```python
from build123d import *

# Parameters (mm, degrees)
F1_DEPTH = 15
F2_R     = 2.125
F3_DEPTH = 18.001
F4_R     = 3.5
F5_DEPTH = 6


with BuildPart() as f1:
    # F0 (on Top) → F1 (new body)
    with BuildSketch(Plane.XY):
        with BuildLine():
            Line((-13.829164, 6.4), (-13.829164, 0))
            Line((-13.829164, 0), (20, 0))
            Line((20, 0), (20, 5))
            Line((20, 5), (10, 5))
            Line((10, 5), (10, 8))
            ThreePointArc((10, 8), (7.071068, 15.071068), (0, 18))
            Line((0, 18), (-13.829164, 18))
            Line((-13.829164, 18), (-13.829164, 9.6))
            Line((-13.829164, 9.6), (-3.829164, 9.6))
            ThreePointArc((-3.829164, 9.6), (4.15, 8), (-3.829164, 6.4))
            Line((-3.829164, 6.4), (-13.829164, 6.4))
        make_face()
    extrude(amount=F1_DEPTH)

    # F2 (on face) → F3 (cut, through all)
    with BuildSketch(Plane.XZ):
        with Locations((-7.5, 7.5)):
            Circle(F2_R)
        with Locations((15, 7.5)):
            Circle(F2_R)
    extrude(amount=-F3_DEPTH, mode=Mode.SUBTRACT)

    # F4 (on face) → F5 (cut)
    with BuildSketch(Plane(origin=(0, 18, 0), x_dir=(-1, 0, 0), z_dir=(0, 1, 0))):
        with Locations((7.5, 7.5)):
            Circle(F4_R)
    extrude(amount=-F5_DEPTH, mode=Mode.SUBTRACT)


solid = f1.part
```
For this review, take the finished solid that the model builds, in its own axes (mm). A direction names the side the tool comes from. Round coordinates to 2 decimals unless told otherwise and drop trailing zeros. Order: outer loops, then holes, each group sorted by start corner. A loop starts at its lowest first (then second) coordinate and runs counter-clockwise, first axis right, second up.
Q1. We need section C-C, the plane x = -7.5. Give the boundary of the cut face in (y, z) (3 decimals), plus the area to 3 significant figures.
Findings below:
outline: (0, 0) - (6.4, 0) - (6.4, 5.375) - (0, 5.375) - close; (0, 9.625) - (6.4, 9.625) - (6.4, 15) - (0, 15) - close; (9.6, 0) - (18, 0) - (18, 4) - (12, 4) - (12, 5.375) - (9.6, 5.375) - close; (9.6, 9.625) - (12, 9.625) - (12, 11) - (18, 11) - (18, 15) - (9.6, 15) - close
area: 143 mm2
Q2. We need section D-D, the plane x = 2. Give the boundary of the cut face in (y, z), plus the area to 3 significant figures.
Findings below:
outline: (0, 0) - (4.36, 0) - (4.36, 15) - (0, 15) - close; (11.64, 0) - (17.8, 0) - (17.8, 15) - (11.64, 15) - close
area: 158 mm2
Q3. Machinability: for faces 1 (the flat face through (-13.829, 14, 7)), 2 (the flat face through (-10, 9.6, 7)), 3 (the flat face through (17.3, 5, 7.4)), 4 (the cylindrical face through (-4.7, 15, 5.4)), which of the approach directions +Z, -Z, +X, -X, +Y, -Y give a long, thin tool a straight path to every point of the face, cutting with its end or side? Answer none if there is none.
Findings below:
face 1: +Z, -Z, -X, +Y, -Y
face 2: +Z, -Z, -X
face 3: +Z, -Z, +X, +Y
face 4: +Y
Q4. We need section A-A, the plane z = 7.5. Give the boundary of the cut face in (x, y) (3 decimals), plus the area to 3 significant figures.
Findings below:
outline: (-13.829, 0) - (-9.625, 0) - (-9.625, 6.4) - (-13.829, 6.4) - close; (-13.829, 9.6) - (-9.625, 9.6) - (-9.625, 12) - (-11, 12) - (-11, 18) - (-13.829, 18) - close; (-5.375, 0) - (12.875, 0) - (12.875, 5) - (10, 5) - (10, 8) arc R10 ccw to (0, 18) - (-4, 18) - (-4, 12) - (-5.375, 12) - (-5.375, 9.6) - (-3.829, 9.6) arc R4.15 cw (long way) to (-3.829, 6.4) - (-5.375, 6.4) - close; (17.125, 0) - (20, 0) - (20, 5) - (17.125, 5) - close
area: 271 mm2
Q5. Wall thickness on line 1 (Z direction, x = -7.5, y = 14.95); line 2 (Y direction, x = 0, z = 7); line 3 (Y direction, x = -5, z = 4): over which ranges is each line inside the solid? List them lowest first.
Findings below:
line 1: z = 0 to 4, 11 to 15
line 2: y = 0 to 3.85, 12.15 to 18
line 3: y = 0 to 6.4, 9.6 to 18
Q6. Mouldability with a two-part tool opening along Y and no side actions: class faces 5 (the flat face through (3, 0, 7)), 6 (the cylindrical face through (4.147, 8.159, 7.395)), 7 (the cylindrical face through (-6.519, 3.155, 5.615)) as pulls with the +Y half, pulls with the -Y half, needs draft (parallel to the pull), parting line crosses it, or undercut.
Findings below:
face 5: pulls with the -Y half
face 6: undercut
face 7: needs draft
Q7. We need section B-B, the plane y = 6. Give the boundary of the cut face in (x, z) (3 decimals).
Findings below:
outline: (-13.829, 0) - (-3.636, 0) - (-3.636, 15) - (-13.829, 15) - close; (3.636, 0) - (10, 0) - (10, 15) - (3.636, 15) - close; hole circle Ø4.25 at (-7.5, 7.5)
Q8. Insertion check: P1, Ø2, axis at y = 9.5, z = 4, coming from the -X side; P2, Ø3.5, axis at x = 15, z = 7.5, coming from the +Y side; P3, Ø5, axis at x = 16, z = 10.5, coming from the +Y side; P4, Ø4, axis at x = 3, z = 3, coming from the +Y side. Each pin has a flat end and moves straight along its axis. Give the tip position at first contact, or say it passes through.
Findings below:
P1: stops at x = -13.83
P2: passes through
P3: stops at y = 5
P4: stops at y = 17.95
